Geometry check sheet. Reference: the model listing, model coordinates, mm. A direction names the side the tool comes from. Coordinates: 2 decimals unless noted, no trailing zeros. Loops run counter-clockwise (first coordinate to the right, second up) from the corner with the lowest first, then second, coordinate; pieces in that order, holes last. Notation, with made-up numbers: (10.5, -33.5) - (33.5, -33.5) arc R21 cw to (33.5, -19.5) - close; hole circle Ø11 at (72, -2). An arc over 180 degrees is marked (long way). One line per item, written item: value.
from build123d import *

# Parameters (mm, degrees)
F0_W     = 11.43
F0_H     = 133.2484
F1_DEPTH = 4.3053
F2_W     = 11.43
F2_H     = 12.573
F3_DEPTH = 2.8702
F7_D     = 2.2606
F8_D     = 2.2606


with BuildPart() as f1:
    # F0 (on Front) → F1 (new body, symmetric)
    with BuildSketch(Plane.XZ):
        Rectangle(F0_W, F0_H)
    extrude(amount=F1_DEPTH, both=True)

    # F2 (on face) → F3 (join)
    with BuildSketch(Plane.XZ.offset(4.3053)):
        Polygon((5.715, 66.6242), (5.715, 54.0512), (37.6988202333, 54.0512), (37.6988202333, 79.1464), (5.715, 79.1464), (-5.715, 79.1464), (-5.715, 66.6242), align=None)
        with Locations((0, 60.3377)):
            Rectangle(F2_W, F2_H)
    extrude(amount=F3_DEPTH)

    # F4: F1 across plane


with BuildPart() as f1_1:
    add(f1.part)
    add(f1.part.mirror(Plane.XZ))

    # F7 (through all)
    with Locations(Plane.XZ.offset(7.1755)):
        with Locations((0.4064, 60.4774)):
            Hole(F7_D / 2)

    # F8 (through all)
    with Locations(Plane.XZ.offset(4.3053)):
        with Locations((0.4064, -60.5028)):
            Hole(F8_D / 2)


solid = f1_1.part
(1) Material ranges on probe 1 along Y at (x, z) = (9.5, 61.5); probe 2 along Z at (x, y) = (1, 1.5); probe 3 along Z at (x, y) = (9, 4.75), recorded low to high. Write a range as from..to.
Reply:
probe 1: -7.18..-4.31, 4.31..7.18
probe 2: -66.62..-61.46, -59.54..59.52, 61.44..66.62
probe 3: 54.05..79.15
(2) Cross-section at C-C on z = 43.5. Record the cut outline in (x, y) (3 decimals).
Reply:
outline: (-5.715, -4.305) - (5.715, -4.305) - (5.715, 4.305) - (-5.715, 4.305) - close
(3) Release check for a two-part mould opening along Y. For faces 1 (the face through (0, 0, 66.624)), 2 (the face through (16, -6, 54.051)), 3 (the face through (16, -7.176, 67)) record: pulls with the +Y half, pulls with the -Y half, needs draft (parallel to the pull), parting line crosses it, or undercut.
Reply:
face 1: undercut
face 2: needs draft
face 3: pulls with the -Y half
(4) Go/stop test with flat-tipped pins: pin 1 Ø12.5 at (x, z) = (-2.5, 5.5) entering from +Y; pin 2 Ø3.5 at (x, z) = (3, -5.5) entering from -Y; pin 3 Ø1 at (y, z) = (2.5, -41.5) entering from +X (3 decimals). Record where each tip stops, or that it passes through.
Reply:
pin 1: y = 4.31
pin 2: y = -4.31
pin 3: x = 5.715
(5) Access from +Z, -Z, +X, -X, +Y, -Y to the whole of each face (thin tool, end or side, straight path). Record for faces 4 (the face through (16, 6, 54.051)), 5 (the face through (-5.715, 0, 7)), 6 (the face through (16, -4.305, 67)), 7 (the face through (0, -4.305, -5)), 8 (the face through (16, -6, 79.146)).
Reply:
face 4: -Z, +X, -X, +Y
face 5: +Z, -Z, -X, +Y, -Y
face 6: +Z, +X
face 7: -Z, +X, -X, -Y
face 8: +Z, +X, -X, +Y, -Y
(6) Cross-section at A-A on x = 23. Record the cut outline in (y, z), and give its area (3 significant figures).
Reply:
outline: (-7.18, 54.05) - (-4.31, 54.05) - (-4.31, 79.15) - (-7.18, 79.15) - close; (4.31, 54.05) - (7.18, 54.05) - (7.18, 79.15) - (4.31, 79.15) - close
area: 144 mm2
(7) Cross-section at B-B on y = -2.25. Record the cut outline in (x, z) (3 decimals), and give its area (4 significant figures).
Reply:
outline: (-5.715, -66.624) - (5.715, -66.624) - (5.715, 66.624) - (-5.715, 66.624) - close; hole circle Ø2.261 at (0.406, -60.503); hole circle Ø2.261 at (0.406, 60.477)
area: 1,515 mm2
